from build123d import *

# Parameters (mm, degrees)
BASE_DEPTH                       = 4
CONG_1_R                         = 3
ENL_V_MAT_EXTRU_1_DEPTH          = 5
ESQUISSE33_R                     = 1.75
PERCAGE_MAIN_DE_DIEU_DEPTH       = 5
ESQUISSE26_R                     = 2
PERCAGE_BUCK_CONVERTER_DEPTH     = 5
ESQUISSE27_R                     = 2
PERCAGE_TEENSY_MOTEUR_DEPTH      = 5
ESQUISSE28_R                     = 1.5
PERCAGE_CARTE_ALIM_DEPTH         = 5
ESQUISSE29_R                     = 2
PERCAGE_RASP_DEPTH               = 5
ESQUISSE32_R                     = 1.75
PERCAGE_TEENSY_ACTIONNEURS_DEPTH = 5
ESQUISSE30_R                     = 2
PERCAGE_ALIM_ACTIONNEURS_DEPTH   = 5
PER_AGE_FILS_DEPTH               = 5
ESQUISSE34_R                     = 1.75
PER_AGE_MOTEUR_ASCENSEUR_DEPTH   = 5
ESQUISSE35_R                     = 1.2
PER_AGE_DRIVER_ASCENSEUR_DEPTH   = 5
ESQUISSE36_R                     = 1.75
ENL_V_MAT_EXTRU_2_DEPTH          = 5
ESQUISSE39_R                     = 2
PER_AGE_EQUERRE_DEPTH            = 5
ESQUISSE38_W                     = 67.748737342
ESQUISSE38_H                     = 31
ENL_V_MAT_EXTRU_3_DEPTH          = 5
CONG_2_R                         = 5


with BuildPart() as part:
    # Esquisse1 → Base (new body)
    with BuildSketch(Plane.XY):
        Polygon((0, 0), (-200, 0), (-224.748737342, 24.748737342), (-224.748737342, 284.748737342), (-200, 309.497474683), (0, 309.497474683), (24.748737342, 284.748737342), (24.748737342, 24.748737342), align=None)
    extrude(amount=BASE_DEPTH)

    # Congé1
    cong_1_edges = [part.edges().sort_by_distance(p)[0] for p in [
        (0, 0, 2),
        (-200, 0, 2),
        (-224.748737342, 24.748737342, 2),
        (-224.748737342, 284.748737342, 2),
        (-200, 309.497474683, 2),
        (0, 309.497474683, 2),
        (24.748737342, 284.748737342, 2),
        (24.748737342, 24.748737342, 2),
    ]]
    fillet(cong_1_edges, radius=CONG_1_R)

    # Esquisse25 → Enlèv. mat.-Extru.1 (cut, through all)
    with BuildSketch(Plane(origin=(0, 0, 0), x_dir=(-1, 0, 0), z_dir=(0, 0, -1))):
        Polygon((-24.748737342, 33), (-24.748737342, 0), (45, 0), (155, 0), (224.748737342, 0), (224.748737342, 33), (224.748737342, 276.497474683), (224.748737342, 309.497474683), (155, 309.497474683), (45, 309.497474683), (-24.748737342, 309.497474683), (-24.748737342, 276.497474683), align=None)
        Polygon((-21.748737342, 33), (45, 33), (45, 3), (155, 3), (155, 33), (221.748737342, 33), (221.748737342, 276.497474683), (155, 276.497474683), (155, 306.497474683), (45, 306.497474683), (45, 276.497474683), (-21.748737342, 276.497474683), align=None, mode=Mode.SUBTRACT)
    extrude(amount=-ENL_V_MAT_EXTRU_1_DEPTH, mode=Mode.SUBTRACT)

    # Esquisse33 → Percage Main_De_Dieu (cut, through all)
    with BuildSketch(Plane.XY.offset(4)):
        with Locations((-207.248737342, 231.748737342)):
            Circle(ESQUISSE33_R)
        with Locations((-187.248737342, 231.748737342)):
            Circle(ESQUISSE33_R)
        with Locations((-207.248737342, 77.748737342)):
            Circle(ESQUISSE33_R)
        with Locations((-187.248737342, 77.748737342)):
            Circle(ESQUISSE33_R)
    extrude(amount=-PERCAGE_MAIN_DE_DIEU_DEPTH, mode=Mode.SUBTRACT)

    # Esquisse26 → Percage Buck Converter (cut, through all)
    with BuildSketch(Plane(origin=(0, 0, 0), x_dir=(-1, 0, 0), z_dir=(0, 0, -1))):
        with Locations((212.748737342, 189.748737342)):
            Circle(ESQUISSE26_R)
        with Locations((212.748737342, 219.748737342)):
            Circle(ESQUISSE26_R)
        with Locations((212.748737342, 89.748737342)):
            Circle(ESQUISSE26_R)
        with Locations((212.748737342, 119.748737342)):
            Circle(ESQUISSE26_R)
    extrude(amount=-PERCAGE_BUCK_CONVERTER_DEPTH, mode=Mode.SUBTRACT)

    # Esquisse27 → Percage Teensy Moteur (cut, through all)
    with BuildSketch(Plane(origin=(0, 0, 0), x_dir=(-1, 0, 0), z_dir=(0, 0, -1))):
        with Locations((142.251262658, 66)):
            Circle(ESQUISSE27_R)
        with Locations((63.251262658, 66)):
            Circle(ESQUISSE27_R)
    extrude(amount=-PERCAGE_TEENSY_MOTEUR_DEPTH, mode=Mode.SUBTRACT)

    # Esquisse28 → Percage Carte Alim (cut, through all)
    with BuildSketch(Plane(origin=(0, 0, 0), x_dir=(-1, 0, 0), z_dir=(0, 0, -1))):
        with Locations((166.748737342, 251.497474683)):
            Circle(ESQUISSE28_R)
        with Locations((102.998737342, 251.497474683)):
            Circle(ESQUISSE28_R)
        with Locations((166.748737342, 169.022474683)):
            Circle(ESQUISSE28_R)
    extrude(amount=-PERCAGE_CARTE_ALIM_DEPTH, mode=Mode.SUBTRACT)

    # Esquisse29 → Percage Rasp (cut, through all)
    with BuildSketch(Plane(origin=(0, 0, 0), x_dir=(-1, 0, 0), z_dir=(0, 0, -1))):
        with Locations((81.748737342, 212.497474683)):
            Circle(ESQUISSE29_R)
        with Locations((23.748737342, 212.497474683)):
            Circle(ESQUISSE29_R)
        with Locations((23.748737342, 261.497474683)):
            Circle(ESQUISSE29_R)
        with Locations((81.748737342, 261.497474683)):
            Circle(ESQUISSE29_R)
    extrude(amount=-PERCAGE_RASP_DEPTH, mode=Mode.SUBTRACT)

    # Esquisse32 → Percage Teensy Actionneurs (cut, through all)
    with BuildSketch(Plane.XY.offset(4)):
        with Locations((-118.251262658, 262.827474683)):
            Circle(ESQUISSE32_R)
        with Locations((-118.251262658, 209.827474683)):
            Circle(ESQUISSE32_R)
        with Locations((-48.111262658, 236.497474683)):
            Circle(ESQUISSE32_R)
    extrude(amount=-PERCAGE_TEENSY_ACTIONNEURS_DEPTH, mode=Mode.SUBTRACT)

    # Esquisse30 → Percage Alim Actionneurs (cut, through all)
    with BuildSketch(Plane(origin=(0, 0, 0), x_dir=(-1, 0, 0), z_dir=(0, 0, -1))):
        with Locations((104.251262658, 133)):
            Circle(ESQUISSE30_R)
        with Locations((58.251262658, 133)):
            Circle(ESQUISSE30_R)
        with Locations((58.251262658, 188.8)):
            Circle(ESQUISSE30_R)
        with Locations((104.251262658, 188.8)):
            Circle(ESQUISSE30_R)
    extrude(amount=-PERCAGE_ALIM_ACTIONNEURS_DEPTH, mode=Mode.SUBTRACT)

    # Esquisse31 → Perçage Fils (cut, through all)
    with BuildSketch(Plane(origin=(0, 0, 0), x_dir=(-1, 0, 0), z_dir=(0, 0, -1))):
        with BuildLine():
            Line((138.251262658, 88), (38.251262658, 88))
            ThreePointArc((38.251262658, 88), (23.251262658, 103), (38.251262658, 118))
            Line((38.251262658, 118), (138.251262658, 118))
            ThreePointArc((138.251262658, 118), (153.251262658, 103), (138.251262658, 88))
        make_face()
    extrude(amount=-PER_AGE_FILS_DEPTH, mode=Mode.SUBTRACT)

    # Esquisse34 → Perçage Moteur Ascenseur (cut, through all)
    with BuildSketch(Plane(origin=(0, 0, 0), x_dir=(-1, 0, 0), z_dir=(0, 0, -1))):
        with Locations((169.623737342, 153.9)):
            Circle(ESQUISSE34_R)
        with Locations((191.873737342, 153.9)):
            Circle(ESQUISSE34_R)
        with Locations((169.623737342, 135.5)):
            Circle(ESQUISSE34_R)
        with Locations((191.873737342, 135.5)):
            Circle(ESQUISSE34_R)
    extrude(amount=-PER_AGE_MOTEUR_ASCENSEUR_DEPTH, mode=Mode.SUBTRACT)

    # Esquisse35 → Perçage Driver Ascenseur (cut, through all)
    with BuildSketch(Plane.XY.offset(4)):
        with Locations((-139.748737342, 149)):
            Circle(ESQUISSE35_R)
        with Locations((-113.748737342, 149)):
            Circle(ESQUISSE35_R)
        with Locations((-113.748737342, 84)):
            Circle(ESQUISSE35_R)
        with Locations((-139.748737342, 84)):
            Circle(ESQUISSE35_R)
    extrude(amount=-PER_AGE_DRIVER_ASCENSEUR_DEPTH, mode=Mode.SUBTRACT)

    # Esquisse36 → Enlèv. mat.-Extru.2 (cut)
    with BuildSketch(Plane.XY.offset(4)):
        with Locations((-155, 194.497474683)):
            Circle(ESQUISSE36_R)
        with Locations((-155, 221.497474683)):
            Circle(ESQUISSE36_R)
    extrude(amount=-ENL_V_MAT_EXTRU_2_DEPTH, mode=Mode.SUBTRACT)

    # Esquisse39 → Perçage Equerre (cut, through all)
    with BuildSketch(Plane.XY.offset(4)):
        with Locations((-145, 286.497474683)):
            Circle(ESQUISSE39_R)
        with Locations((-165, 266.497474683)):
            Circle(ESQUISSE39_R)
        with Locations((-35, 266.497474683)):
            Circle(ESQUISSE39_R)
        with Locations((-55, 286.497474683)):
            Circle(ESQUISSE39_R)
        with Locations((-35, 43)):
            Circle(ESQUISSE39_R)
        with Locations((-55, 23)):
            Circle(ESQUISSE39_R)
        with Locations((-165, 43)):
            Circle(ESQUISSE39_R)
        with Locations((-145, 23)):
            Circle(ESQUISSE39_R)
    extrude(amount=-PER_AGE_EQUERRE_DEPTH, mode=Mode.SUBTRACT)

    # Esquisse38 → Enlèv. mat.-Extru.3 (cut, through all)
    with BuildSketch(Plane(origin=(0, 0, 0), x_dir=(-1, 0, 0), z_dir=(0, 0, -1))):
        with Locations((12.125631329, 18.5)):
            Rectangle(ESQUISSE38_W, ESQUISSE38_H)
        with Locations((187.874368671, 18.5)):
            Rectangle(ESQUISSE38_W, ESQUISSE38_H)
        with Locations((187.874368671, 290.997474683)):
            Rectangle(ESQUISSE38_W, ESQUISSE38_H)
        with Locations((12.125631329, 290.997474683)):
            Rectangle(ESQUISSE38_W, ESQUISSE38_H)
    extrude(amount=-ENL_V_MAT_EXTRU_3_DEPTH, mode=Mode.SUBTRACT)

    # Congé2
    cong_2_edges = [part.edges().sort_by_distance(p)[0] for p in [
        (21.748737342, 275.497474683, 2),
        (-46, 306.497474683, 2),
        (-221.748737342, 275.497474683, 2),
        (-154, 306.497474683, 2),
        (-221.748737342, 34, 2),
        (-154, 3, 2),
        (21.748737342, 34, 2),
        (-46, 3, 2),
    ]]
    fillet(cong_2_edges, radius=CONG_2_R)


solid = part.part
Design review of the part built by this model. Coordinates are the model's own, in mm. A direction names the side the tool comes from. Coordinates: 2 decimals unless noted, no trailing zeros. Order: outer loops, then holes, each group sorted by start corner. A loop starts at its lowest first (then second) coordinate and runs counter-clockwise, first axis right, second up.
Item 1: For faces 1 (the flat face through (-98, 157, 4)), 2 (the cylindrical face through (-23.255, 102.67, 1.972)), list the 3-axis set-ups (+Z, -Z, +X, -X, +Y, -Y) from which the entire face can be reached by the end or side of a thin tool; tool diameter is ignored.
Item 2: Take a section at C-C, the plane z = 1.15. Count the separate pieces of the cut face and the enclosed holes in it, then the cut area to 3 significant figures.
Item 3: For pin 1 Ø2.5 at (x, y) = (-58.25, 188.8) entering from +Z, flat-tipped, find the tip position at first contact; note if it passes through.
Item 4: Take a section at A-A, the plane x = -89. Write out the cut boundary in (y, z).
Item 5: Take a section at D-D, the plane x = -1.5. Write out the cut boundary in (y, z).
Item 6: Take a section at B-B, the plane y = 103. Write out the cut boundary in (x, z), then the cut area to 3 significant figures.
Item 7: For line 1 (X direction, y = 84, z = 2.6); line 2 (Y direction, x = -207.5, z = 3.75); line 3 (Y direction, x = -55, z = 3.3), list the stretches that pass through material, from the lowest coordinate up.
Item 8: The part is to be moulded in two halves that separate along Y. For faces 3 (the flat face through (-98, 157, 0)), 4 (the cylindrical face through (-153.248, 103.33, 1.972)), say which applies: pulls with the +Y half, pulls with the -Y half, needs draft (parallel to the pull), parting line crosses it, or undercut.
The answers:
1. face 1: +Z, +X, -X, +Y, -Y
1. face 2: +Z, -Z
2. separate pieces: 1
2. enclosed holes: 43
2. area: 61,300 mm2
3. pin 1: passes through
4. outline: (3, 0) - (88, 0) - (88, 4) - (3, 4) - close; (118, 0) - (306.5, 0) - (306.5, 4) - (118, 4) - close
5. outline: (34, 0) - (275.5, 0) - (275.5, 4) - (34, 4) - close
6. outline: (-221.75, 0) - (-153.25, 0) - (-153.25, 4) - (-221.75, 4) - close; (-23.25, 0) - (21.75, 0) - (21.75, 4) - (-23.25, 4) - close
6. area: 454 mm2
7. line 1: x = -221.75 to -140.95, -138.55 to -114.95, -112.55 to 21.75
7. line 2: y = 34 to 76.02, 79.48 to 230.02, 233.48 to 275.5
7. line 3: y = 3 to 21, 25 to 88, 118 to 284.5, 288.5 to 306.5
8. face 3: needs draft
8. face 4: undercut
